Autodesk Fusion 360 part; units mm, degrees
sketch "Sketch1" plane through (0, 0, 0) normal (0, 1, 0) x (1, 0, 0)
  line L0 (0, 0) -> (62.5, 0)
  line L1 (62.5, 0) -> (62.5, -5)
  line L2 (62.5, -5) -> (52.5, -5)
  arc A0 (52.5, -5) -> (43.75, -11.5668) centre (52.5, -14.1129) ccw
  line L3 (43.75, -11.5668) -> (38.15, -30.812)
  arc A1 (24.35, -30.812) -> (38.15, -30.812) centre (31.25, -23.3) ccw
  line L4 (24.35, -30.812) -> (18.75, -11.5668)
  arc A2 (18.75, -11.5668) -> (10, -5) centre (10, -14.1129) ccw
  line L5 (10, -5) -> (0, -5)
  line L6 (0, -5) -> (0, 0)
  circle A3 centre (31.25, -23.3) radius 2.5
  line L7 (24.35, -30.812) -> (38.15, -30.812) construction
  line L8 (31.25, -33.5) -> (31.25, -23.3) construction
  line L9 (10, -5) -> (52.5, -5)
  dimension "d1" = 13.8
  dimension "d2" = 7.7
  dimension "d3" = 5
  dimension "d5" = 5
  dimension "d8" = 62.5
  dimension "d29" = 33.5
  dimension "d30" = 25
  dimension "d31" = 10
extrude "Extrude1" add sketch "Sketch1" along normal blind 6
extrude "Extrude2" add sketch "Sketch1" against normal blind 10 contours L0 L1 L2 L5 L6 L9
extrude "Extrude3" add 1 faces at (31.3123, 6, 14.6469) along direction (0, -1, 0) blind 6 from surface at 16
fillet "Fillet1" radius 1 4 edges at (0, -16, 2.5) (62.5, -16, 2.5) (62.5, 6, 2.5) (0, 6, 2.5)
sketch "Sketch2" plane through (0, 0, 0) normal (0, 0, -1) x (1, 0, 0)
  arc A0 (0, -5) -> (1, -6) centre (1, -5) ccw
  line L0 (1, -6) -> (61.5, -6)
  arc A1 (61.5, -6) -> (62.5, -5) centre (61.5, -5) ccw
  line L1 (62.5, -5) -> (62.5, 15)
  arc A2 (62.5, 15) -> (61.5, 16) centre (61.5, 15) ccw
  line L2 (61.5, 16) -> (1, 16)
  arc A3 (1, 16) -> (0, 15) centre (1, 15) ccw
  line L3 (0, 15) -> (0, -5)
  line L4 (0, 5) -> (62.5, 5) construction
  circle A4 centre (11, 5) radius 2.5
  circle A5 centre (51.5, 5) radius 2.5
  line L5 (31.25, 5) -> (31.25, 16) construction
  dimension "d20" = 40.5
  dimension "d21" = 5
extrude "Extrude4" cut sketch "Sketch2" against normal blind 7 contours A4 | A5
chamfer "Chamfer1" distance 2 angle 45 2 edges at (8.6692, -4.096, 5) (49.1692, -4.096, 5)
chamfer "Chamfer2" distance 0.5 angle 45 27 edges at (40.95, 6, 21.1894) (47.03, 6, 6.8243) (57, 6, 5) (62.2071, 5.7071, 5) (62.5, -5, 5) (62.2071, -15.7071, 5) (57, -16, 5) (47.03, -16, 6.8243) (40.95, -16, 21.1894) (21.55, 6, 21.1894) (21.55, -16, 21.1894) (15.47, -16, 6.8243) (5.5, -16, 5) (0.2929, -15.7071, 5) (0, -5, 5) (0.2929, 5.7071, 5) (5.5, 6, 5) (15.47, 6, 6.8243) (31.25, 6, 33.5) (31.25, 6, 0) (0.2929, 5.7071, 0) (0, -5, 0) (0.2929, -15.7071, 0) (31.25, -16, 0) (62.2071, -15.7071, 0) (62.5, -5, 0) (62.2071, 5.7071, 0)
fillet "Fillet3" radius 0.5 2 edges at (31.25, -10, 5) (31.25, 0, 5)
Design review of the part built by this model. Coordinates are the model's own, in mm. A direction names the side the tool comes from. Round coordinates to 2 decimals unless told otherwise and drop trailing zeros. Write each loop counter-clockwise with the first axis right and the second up, starting at its lowest first coordinate (ties: lowest second). Pieces come first, ordered by that corner, then holes. Notation, with made-up numbers: (-2.75, -7) -> (11.25, -7) arc R16 cw to (11.25, 14) -> close; hole circle Ø7 at (77, 62.5). An arc over 180 degrees is marked (long way). One line per question, with ' | ' between items.
(1) Machinability: for faces 1 (the conical face through (15.489, -15.642, 6.661)), 2 (the flat face through (31, -10, 16)), which of the approach directions +Z, -Z, +X, -X, +Y, -Y give a long, thin tool a straight path to every point of the face, cutting with its end or side? Answer none if there is none.
Result sheet:
face 1: +Z, -X, -Y | face 2: +Z, +X, -X
(2) Take a section at A-A, the plane y = -5. State the section outline as (x, z) points.
Result sheet:
outline: (0, 0.5) -> (0.5, 0) -> (8.5, 0) -> (8.5, 3) -> (6.5, 5) -> (0.5, 5) -> (0, 4.5) -> close; (13.5, 0) -> (49, 0) -> (49, 3) -> (47, 5) -> (15.5, 5) -> (13.5, 3) -> close; (54, 0) -> (62, 0) -> (62.5, 0.5) -> (62.5, 4.5) -> (62, 5) -> (56, 5) -> (54, 3) -> close
(3) Draft analysis for pull direction Y (two halves, no side actions). For faces 3 (the flat face through (31, -5, 0)), 4 (the conical face through (15.62, 5.64, 6.76)), 5 (the conical face through (13.504, -4.211, 3.125)), state which applies: released by +Y, released by -Y, zero draft, split by the parting line, or undercut.
Result sheet:
face 3: zero draft | face 4: released by +Y | face 5: undercut
(4) Wall thickness on line 1 (X direction, y = -5, z = 1.55); line 2 (Y direction, x = 38.5, z = 16); line 3 (Y direction, x = 11, z = 2.3): over which ranges is each line inside the solid? List them lowest first. Write a range as [from, to].
Result sheet:
line 1: [0, 8.5], [13.5, 49], [54, 62.5] | line 2: [-16, -10], [0, 6] | line 3: [-16, -7.5], [-2.5, 6]
(5) Insertion check: P1, Ø10.5, axis at x = 42, y = -8.5, coming from the +Z side; P2, Ø10, axis at x = 41, y = 0.5, coming from the +Z side; P3, Ø10, axis at x = 39.5, y = 3.5, coming from the +Z side. Each pin has a flat end and moves straight along its axis. Give the tip position at first contact, or say it passes through.
Result sheet:
P1: z = 31.75 | P2: z = 32.33 | P3: z = 32.97
(6) Take a section at D-D, the plane y = 2. State the section outline as (x, z) points.
Result sheet:
outline: (0, 0.5) -> (0.5, 0) -> (62, 0) -> (62.5, 0.5) -> (62.5, 4.5) -> (62, 5) -> (52.5, 5) arc R9.11 cw to (43.75, 11.57) -> (38.15, 30.81) arc R10.2 ccw to (24.35, 30.81) -> (18.75, 11.57) arc R9.11 cw to (10, 5) -> (0.5, 5) -> (0, 4.5) -> close; hole circle Ø5 at (31.25, 23.3)
(7) Take a section at B-B, the plane x = 5. State the section outline as (y, z) points.
Result sheet:
outline: (-16, 0.5) -> (-15.5, 0) -> (5.5, 0) -> (6, 0.5) -> (6, 4.5) -> (5.5, 5) -> (-15.5, 5) -> (-16, 4.5) -> close
(8) Take a section at C-C, the plane z = 29.5. State the section outline as (x, y) points, and give its area (3 significant figures).
Result sheet:
outline: (23.97, -15.5) -> (24.49, -16) -> (38.01, -16) -> (38.53, -15.5) -> (38.53, -10) -> (23.97, -10) -> close; (23.97, 0) -> (38.53, 0) -> (38.53, 5.5) -> (38.01, 6) -> (24.49, 6) -> (23.97, 5.5) -> close | area: 174 mm2
